Model file for the job. Use its own axes, mm. Face numbers are marked on the shaded views. A direction names the side the tool comes from. Round coordinates to 2 decimals unless told otherwise and drop trailing zeros. Write each loop counter-clockwise with the first axis right and the second up, starting at its lowest first coordinate (ties: lowest second). Pieces come first, ordered by that corner, then holes.
```python
from build123d import *

# Parameters (mm, degrees)
EXTRUDE_1_DEPTH      = 6
CHAMFER_1_SIZE       = 4
SKETCH_2_R           = 1.5
CUT_EXTRUDE_1_DEPTH  = 63.816723883
EXTRUDE_2_DEPTH      = 4
EXTRUDE_2_DEPTH_BACK = 10
CHAMFER_2_SIZE       = 4


with BuildPart() as part:
    # 草图1 → 凸台-拉伸1 (new body)
    with BuildSketch(Plane.XY):
        with BuildLine():
            Line((-5, 0), (-5, 25.056196909))
            Line((-5, 25.056196909), (-17.757675909, 56.63255283))
            Line((-17.757675909, 56.63255283), (-8.485837363, 60.378618764))
            Line((-8.485837363, 60.378618764), (-4.739771429, 51.106780219))
            Line((-4.739771429, 51.106780219), (-7.577195414, 44.422228211))
            Line((-7.577195414, 44.422228211), (-2.08588611, 31.544125784))
            Line((-2.08588611, 31.544125784), (4.250786813, 28.854367709))
            Line((4.250786813, 28.854367709), (5, 27))
            Line((5, 27), (5, 0))
            ThreePointArc((5, 0), (0, -5), (-5, 0))
        make_face()
    extrude(amount=EXTRUDE_1_DEPTH)

    # 倒角1
    chamfer_1_edges = [part.edges().sort_by_distance(p)[0] for p in [
        (-17.757675909, 56.63255283, 3),
    ]]
    chamfer(chamfer_1_edges, length=CHAMFER_1_SIZE)

    # 草图2 → 切除-拉伸1 (cut, through all)
    with BuildSketch(Plane.XY.offset(6)):
        with Locations((0, 27.08857665)):
            Circle(SKETCH_2_R)
        Circle(SKETCH_2_R)
    extrude(amount=-CUT_EXTRUDE_1_DEPTH, mode=Mode.SUBTRACT)

    # 草图3 → 凸台-拉伸2 (add, two sides: drawn at the far end of the back side and taken through both)
    with BuildSketch(Plane(origin=(0, 0, 0), x_dir=(-1, 0, 0), z_dir=(0, 0, -1)).offset(-EXTRUDE_2_DEPTH_BACK)):
        Polygon((16.259249535, 52.923817412), (14.04894049, 58.130979204), (8.485837363, 60.378618764), (4.739771429, 51.106780219), (7.577195414, 44.422228211), (12.088045963, 42.599726288), align=None)
    extrude(amount=EXTRUDE_2_DEPTH + EXTRUDE_2_DEPTH_BACK)

    # 倒角2
    chamfer_2_edges = [part.edges().sort_by_distance(p)[0] for p in [
        (-9.832620688, 43.51097725, 6),
        (-9.832620688, 43.51097725, 0),
    ]]
    chamfer(chamfer_2_edges, length=CHAMFER_2_SIZE - 0.0001)  # a hair under: the kernel refuses the full size


solid = part.part
```
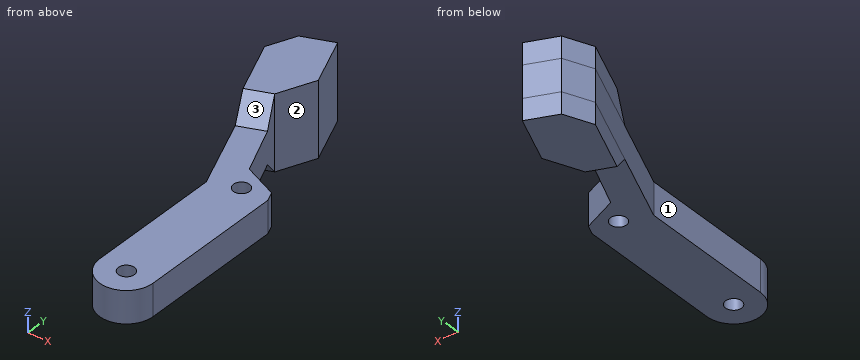
1) Cut at D-D on z = -1. List the corners of the cut face in (x, y).
2) Flat gauge pins, fed straight in: pin 1 Ø12.5 at (x, y) = (1, 29) entering from -Z; pin 2 Ø1 at (x, z) = (-1.5, 5) entering from +Y; pin 3 Ø2.5 at (x, y) = (0, 0) entering from -Z; pin 4 Ø5 at (y, z) = (12, 8) entering from +X. Where does each tip first touch, or does it go through?
3) Cut at A-A on x = 0. List the corners of the cut face in (y, z).
4) Which spindle directions (+Z, -Z, +X, -X, +Y, -Y) get a long thin tool onto all of the face, cutting with end or side? Do the marked faces 1, 2 and 3. Say none if no direction does.
5) Cut at C-C on y = 2.5. List the corners of the cut face in (x, z).
6) Cut at B-B on z = 4.5. List the corners of the cut face in (x, y).
7) Wall check: probe 1 along Y at (x, z) = (0, 2.35); probe 2 along Y at (x, z) = (-1.25, 2.75); probe 3 along Z at (x, y) = (0.5, 24). Give the ranges that are in metal, low to high.
Result sheet:
1. outline: (-16.26, 52.92) - (-10.96, 39.82) - (-6.4, 41.66) - (-7.58, 44.42) - (-4.74, 51.11) - (-8.49, 60.38) - (-14.05, 58.13) - close
2. pin 1: stops at z = 0
2. pin 2: stops at y = 31.51
2. pin 3: passes through
2. pin 4: stops at x = 5
3. outline: (-5, 0) - (-1.5, 0) - (-1.5, 6) - (-5, 6) - close; (1.5, 0) - (25.59, 0) - (25.59, 6) - (1.5, 6) - close; (28.59, 0) - (30.66, 0) - (30.66, 6) - (28.59, 6) - close
4. face 1: +Z, -Z, -X, -Y
4. face 2: +Z, -Z, +X
4. face 3: +Z, +X, -Y
5. outline: (-5, 0) - (5, 0) - (5, 6) - (-5, 6) - close
6. outline: (-16.26, 52.92) - (-5, 25.06) - (-5, 0) arc R5 ccw to (5, 0) - (5, 27) - (4.25, 28.85) - (-2.09, 31.54) - (-7.58, 44.42) - (-4.74, 51.11) - (-8.49, 60.38) - (-14.05, 58.13) - close; hole circle Ø3 at (0, 0); hole circle Ø3 at (0, 27.09)
7. probe 1: y = -5 to -1.5, 1.5 to 25.59, 28.59 to 30.66
7. probe 2: y = -4.84 to -0.83, 0.83 to 26.26, 27.92 to 31.19
7. probe 3: z = 0 to 6
